from build123d import *

# Parameters (mm, degrees)
BOSS_EXTRUDE1_DEPTH      = 55.88
BOSS_EXTRUDE1_DEPTH_BACK = 25.384918905
SKETCH1_W                = 107.698417182
SKETCH1_H                = 40.435670154
SKETCH7_W                = 43.633869471
SKETCH7_H                = 43.18
CUT_EXTRUDE8_DEPTH       = 88.506314553
SKETCH11_R               = 5.08
CUT_EXTRUDE9_DEPTH       = 100.561464261
FILLET2_R                = 2.54
SKETCH13_W               = 44.238094174
SKETCH13_H               = 45.644522424
CUT_EXTRUDE12_DEPTH      = 88.506314553
SKETCH16_W               = 19.145212778
SKETCH16_H               = 40.435670154
BOSS_EXTRUDE3_DEPTH      = 19.05
SKETCH17_W               = 18.93986558
SKETCH17_H               = 40.435670154
BOSS_EXTRUDE4_DEPTH      = 19.05
SKETCH18_R               = 5.08
CUT_EXTRUDE14_DEPTH      = 101.743662762
SKETCH19_W               = 12.523537134
SKETCH19_H               = 13.59850093
SKETCH19_W_2             = 10.108917538
SKETCH19_H_2             = 12.59254748
CUT_EXTRUDE15_DEPTH      = 19.05
SKETCH20_W               = 18.93986558
SKETCH20_H               = 22.510158117
CUT_EXTRUDE16_DEPTH      = 12.7
SKETCH23_W               = 22.632454672
SKETCH23_H               = 12.59254748
CUT_EXTRUDE19_DEPTH      = 12.7
SKETCH24_W               = 19.174620912
SKETCH24_H               = 22.632454672
CUT_EXTRUDE20_DEPTH      = 12.7
FILLET4_R                = 2.54
FILLET5_R                = 2.54
SKETCH25_W               = 8.617694519
SKETCH25_H               = 43.18
BOSS_EXTRUDE5_DEPTH      = 6.35
SKETCH26_W               = 8.674470407
SKETCH26_H               = 43.18
BOSS_EXTRUDE6_DEPTH      = 6.35
SKETCH27_R               = 2.5
CUT_EXTRUDE21_DEPTH      = 6.35
SKETCH22_W               = 22.632454672
SKETCH22_H               = 12.59254748
CUT_EXTRUDE18_DEPTH      = 12.7


with BuildPart() as part:
    # Sketch1 → Boss-Extrude1 (new, two sides: drawn at the far end of the back side and taken through both)
    with BuildSketch(Plane(origin=(0, 0, 0), x_dir=(1, 0, 0), z_dir=(0, 1, 0)).offset(-BOSS_EXTRUDE1_DEPTH_BACK)):
        Rectangle(SKETCH1_W, SKETCH1_H)
    extrude(amount=BOSS_EXTRUDE1_DEPTH + BOSS_EXTRUDE1_DEPTH_BACK)

    # Sketch7 → Cut-Extrude8 (cut, through all)
    with BuildSketch(Plane.XY.offset(20.217835077)):
        with Locations((-22.071539031, 15.247540547)):
            Rectangle(SKETCH7_W, SKETCH7_H)
    extrude(amount=-CUT_EXTRUDE8_DEPTH, mode=Mode.SUBTRACT)

    # Sketch11 → Cut-Extrude9 (cut, through all)
    with BuildSketch(Plane(origin=(0, -25.384918905, 0), x_dir=(-1, 0, 0), z_dir=(0, -1, 0))):
        with Locations(Location((-33.631373514, 0, 0), (0, 0, 90))):
            Circle(SKETCH11_R)
    extrude(amount=-CUT_EXTRUDE9_DEPTH, mode=Mode.SUBTRACT)

    # Fillet2
    fillet2_edges = [part.edges().sort_by_distance(p)[0] for p in [
        (53.849208591, 15.247540547, 20.217835077),
        (53.849208591, 15.247540547, -20.217835077),
    ]]
    fillet(fillet2_edges, radius=FILLET2_R)

    # Sketch13 → Cut-Extrude12 (cut, through all)
    with BuildSketch(Plane.XY.offset(20.217835077)):
        with Locations((35.328255678, 12.741509062)):
            Rectangle(SKETCH13_W, SKETCH13_H)
    extrude(amount=-CUT_EXTRUDE12_DEPTH, mode=Mode.SUBTRACT)

    # Sketch16 → Boss-Extrude3 (add)
    with BuildSketch(Plane(origin=(0, 55.88, 0), x_dir=(1, 0, 0), z_dir=(0, 1, 0))):
        with Locations((-44.276602202, 0)):
            Rectangle(SKETCH16_W, SKETCH16_H)
    extrude(amount=BOSS_EXTRUDE3_DEPTH)

    # Sketch17 → Boss-Extrude4 (add)
    with BuildSketch(Plane.XZ.offset(25.384918905)):
        with Locations((-44.379275801, 0)):
            Rectangle(SKETCH17_W, SKETCH17_H)
    extrude(amount=BOSS_EXTRUDE4_DEPTH)

    # Sketch18 → Cut-Extrude14 (cut, through all)
    with BuildSketch(Plane.XY.offset(20.217835077)):
        with Locations((-44.558869733, 65.07512608)):
            Circle(SKETCH18_R)
        with Locations((-44.558869733, -34.785392183)):
            Circle(SKETCH18_R)
    extrude(amount=-CUT_EXTRUDE14_DEPTH, mode=Mode.SUBTRACT)

    # Sketch19 → Cut-Extrude15 (cut)
    with BuildSketch(Plane.ZY.offset(53.849208591)):
        with Locations((-6.261768567, -37.63566844)):
            Rectangle(SKETCH19_W, SKETCH19_H)
        with Locations((5.054458769, -37.63566844)):
            Rectangle(SKETCH19_W_2, SKETCH19_H)
        with Locations((-6.261768567, 68.63372626)):
            Rectangle(SKETCH19_W, SKETCH19_H_2)
        with Locations((5.054458769, 68.63372626)):
            Rectangle(SKETCH19_W_2, SKETCH19_H_2)
    extrude(amount=-CUT_EXTRUDE15_DEPTH, mode=Mode.SUBTRACT)

    # Sketch20 → Cut-Extrude16 (cut)
    with BuildSketch(Plane(origin=(0, -30.836417975, 0), x_dir=(-1, 0, 0), z_dir=(0, -1, 0))):
        with Locations((44.379275801, 1.268458076)):
            Rectangle(SKETCH20_W, SKETCH20_H)
    extrude(amount=-CUT_EXTRUDE16_DEPTH, mode=Mode.SUBTRACT)

    # Sketch23 → Cut-Extrude19 (cut)
    with BuildSketch(Plane.ZY.offset(34.799208591)):
        with Locations((-1.207309798, 68.63372626)):
            Rectangle(SKETCH23_W, SKETCH23_H)
    extrude(amount=-CUT_EXTRUDE19_DEPTH, mode=Mode.SUBTRACT)

    # Sketch24 → Cut-Extrude20 (cut)
    with BuildSketch(Plane(origin=(0, 62.33745252, 0), x_dir=(1, 0, 0), z_dir=(0, 1, 0))):
        with Locations((-44.261898135, 1.207309798)):
            Rectangle(SKETCH24_W, SKETCH24_H)
    extrude(amount=-CUT_EXTRUDE20_DEPTH, mode=Mode.SUBTRACT)

    # Fillet4
    fillet4_edges = [part.edges().sort_by_distance(p)[0] for p in [
        (-44.276602202, 74.93, -12.523537134),
        (-0.254604295, 15.247540547, -20.217835077),
    ]]
    fillet(fillet4_edges, radius=FILLET4_R)

    # Fillet5
    fillet5_edges = [part.edges().sort_by_distance(p)[0] for p in [
        (-34.909343011, -25.384918905, -1.268458075),
        (-34.674587679, 55.88, -1.207309798),
    ]]
    fillet(fillet5_edges, radius=FILLET5_R)

    # Sketch25 → Boss-Extrude5 (add)
    with BuildSketch(Plane.XY.offset(20.217835077)):
        with Locations((-4.563451555, 15.247540547)):
            Rectangle(SKETCH25_W, SKETCH25_H)
    extrude(amount=-BOSS_EXTRUDE5_DEPTH)

    # Sketch26 → Boss-Extrude6 (add)
    with BuildSketch(Plane.XY.offset(20.217835077)):
        with Locations((-39.551238563, 15.247540547)):
            Rectangle(SKETCH26_W, SKETCH26_H)
    extrude(amount=-BOSS_EXTRUDE6_DEPTH)

    # Sketch27 → Cut-Extrude21 (cut)
    with BuildSketch(Plane(origin=(0, 0, 13.867835077), x_dir=(-1, 0, 0), z_dir=(0, 0, -1))):
        with Locations((5.557905154, -1.039158594)):
            Circle(SKETCH27_R)
        with Locations((5.557905154, 31.534239688)):
            Circle(SKETCH27_R)
        with Locations((38.585172907, -1.039158594)):
            Circle(SKETCH27_R)
        with Locations((38.585172907, 31.534239688)):
            Circle(SKETCH27_R)
    extrude(amount=-CUT_EXTRUDE21_DEPTH, mode=Mode.SUBTRACT)

    # Sketch22 → Cut-Extrude18 (cut)
    with BuildSketch(Plane.ZY.offset(34.799208591)):
        with Locations((-1.207309798, 68.63372626)):
            Rectangle(SKETCH22_W, SKETCH22_H)
    extrude(amount=-CUT_EXTRUDE18_DEPTH, mode=Mode.SUBTRACT)


solid = part.part
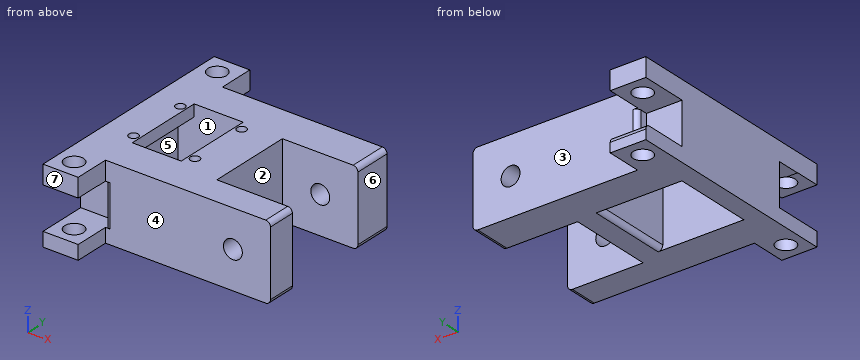
Could you check a few things on this model? Use its own coordinates, in mm. Face numbers are marked on the shaded views. A direction names the side the tool comes from. Coordinates: 2 decimals unless noted, no trailing zeros. Loops run counter-clockwise (first coordinate to the right, second up) from the corner with the lowest first, then second, coordinate; pieces in that order, holes last. Notation, with made-up numbers: (-27, 60) -> (24, 60) arc R26 ccw to (24, 93) -> close; hole circle Ø3 at (48, 46.5). An arc over 180 degrees is marked (long way). Answer in a Markdown table with one row per item.
(1) Imagine slicing it at C-C (x = 31). List the corners of the cut face in (y, z) for me.
Results found:
| item | result |
|---|---|
| outline | (-25.38, -20.22) -> (-10.08, -20.22) -> (-10.08, -4.35) -> (-25.38, -4.35) -> close; (-25.38, 4.35) -> (-10.08, 4.35) -> (-10.08, 20.22) -> (-25.38, 20.22) -> close; (35.56, -20.22) -> (55.88, -20.22) -> (55.88, -4.35) -> (35.56, -4.35) -> close; (35.56, 4.35) -> (55.88, 4.35) -> (55.88, 20.22) -> (35.56, 20.22) -> close |
(2) Imagine slicing it at A-A (y = 58). List the corners of the cut face in (x, z) for me.
Results found:
| item | result |
|---|---|
| outline | (-53.85, -20.22) -> (-34.7, -20.22) -> (-34.7, -12.52) -> (-53.85, -12.52) -> close; (-53.85, 10.11) -> (-34.7, 10.11) -> (-34.7, 20.22) -> (-53.85, 20.22) -> close |
(3) For the marked faces 1, 2, 3 and 4, which set-ups out of +Z, -Z, +X, -X, +Y, -Y let a thin tool reach every point of the face, with its end or its side?
Results found:
| item | result |
|---|---|
| face 1 | -Z |
| face 2 | +Z, -Z, +X |
| face 3 | +Z, -Z, +X, +Y |
| face 4 | +Z, -Z, +X, -Y |
(4) Imagine slicing it at B-B (z = 0). List the corners of the cut face in (x, y) for me, plus the area to 3 significant figures.
Results found:
| item | result |
|---|---|
| outline | (-53.85, -18.14) -> (-34.91, -18.14) -> (-34.91, -22.84) arc R2.54 ccw to (-32.37, -25.38) -> (28.55, -25.38) -> (28.55, -10.08) -> (13.21, -10.08) -> (13.21, 35.56) -> (28.55, 35.56) -> (28.55, 55.88) -> (-32.13, 55.88) arc R2.54 ccw to (-34.67, 53.34) -> (-34.67, 49.64) -> (-53.85, 49.64) -> close; (38.71, -25.38) -> (53.85, -25.38) -> (53.85, -10.08) -> (38.71, -10.08) -> close; (38.71, 35.56) -> (53.85, 35.56) -> (53.85, 55.88) -> (38.71, 55.88) -> close; hole (-43.89, -6.34) -> (-0.25, -6.34) -> (-0.25, 36.84) -> (-43.89, 36.84) -> close |
| area | 4,390 mm^2 |
(5) Will these pins go through, and if not, where does the flat tip stop? pin 1 Ø6.5 at (x, y) = (-38.59, -1.04) entering from +Z; pin 2 Ø21 at (x, z) = (-47.5, -1) entering from +Y; pin 3 Ø8 at (x, y) = (-44.56, -34.79) entering from -Z; pin 4 Ø3 at (y, z) = (51.5, -2.5) entering from -X.
Results found:
| item | result |
|---|---|
| pin 1 | stops at z = 20.22 |
| pin 2 | stops at y = 49.64 |
| pin 3 | passes through |
| pin 4 | stops at x = -34.67 |
(6) If I drill on probe 1 along X at (y, z) = (-1, 2); probe 2 along Y at (x, z) = (19, -3); probe 3 along Y at (x, z) = (-46, 17.5), over which ranges is the centre line in solid material (lowest first)?
Results found:
| item | result |
|---|---|
| probe 1 | x = -53.85 to -43.89, -0.25 to 13.21 |
| probe 2 | y = -25.38 to -10.08, 35.56 to 55.88 |
| probe 3 | y = -44.43 to -39.66, -29.91 to 60.2, 69.95 to 74.93 |
(7) Imagine slicing it at D-D (y = -19.5). List the corners of the cut face in (x, z) for me, plus the area to 3 significant figures.
Results found:
| item | result |
|---|---|
| outline | (-53.85, -20.22) -> (51.31, -20.22) arc R2.54 ccw to (53.85, -17.68) -> (53.85, 17.68) arc R2.54 ccw to (51.31, 20.22) -> (-53.85, 20.22) -> (-53.85, 9.99) -> (-34.91, 9.99) -> (-34.91, -12.52) -> (-53.85, -12.52) -> close; hole circle Ø10.16 at (33.63, 0) |
| area | 3,840 mm^2 |
(8) Thinking about a two-plate mould opening in X: for the marked faces 5, 6 and 7, which applies, released by +X, released by -X, zero draft, split by the parting line, or undercut?
Results found:
| item | result |
|---|---|
| face 5 | undercut |
| face 6 | released by +X |
| face 7 | zero draft |
